Input: part model. Units: mm. Frame: model coordinates. A direction names the side the tool comes from. Give positions to 0.01 mm unless a question says otherwise; leave off trailing zeros. Write each loop counter-clockwise with the first axis right and the second up, starting at its lowest first coordinate (ties: lowest second). Pieces come first, ordered by that corner, then holes.
```python
from build123d import *

# Parameters (mm, degrees)
SKETCH_R        = 13
PAD_DEPTH       = 4
SKETCH001_R     = 11.2
SKETCH001_R_2   = 6.8
POCKET_DEPTH    = 0.5
SKETCH002_R     = 5
POCKET001_DEPTH = 8.001


with BuildPart() as part:
    # Sketch → Pad (new body, symmetric)
    with BuildSketch(Plane.XZ):
        Circle(SKETCH_R)
    extrude(amount=PAD_DEPTH, both=True)

    # Sketch001 (on Face2 of Pad) → Pocket (cut)
    with BuildSketch(Plane(origin=(0, 4, 0), x_dir=(1, 0, 0), z_dir=(0, 1, 0))):
        Circle(SKETCH001_R)
        Circle(SKETCH001_R_2, mode=Mode.SUBTRACT)
    pocket = extrude(amount=-POCKET_DEPTH, mode=Mode.SUBTRACT)

    # Mirrored: Pocket across XZ
    add(pocket.mirror(Plane.XZ), mode=Mode.SUBTRACT)

    # Sketch002 (on Face10 of Mirrored) → Pocket001 (cut, through all)
    with BuildSketch(Plane(origin=(0, 4, 0), x_dir=(1, 0, 0), z_dir=(0, 1, 0))):
        Circle(SKETCH002_R)
    extrude(amount=-POCKET001_DEPTH, mode=Mode.SUBTRACT)


solid = part.part
```
Item 1: Section B-B (z = 0). Return loops of the section in (x, y).
Item 2: Pin query (flat end, axial travel): pin 1 (5 mm diameter, centred on x = -0.5, z = 4, fed in from +Y); pin 2 (3 mm diameter, centred on y = 0.5, z = -7, fed in from +X); pin 3 (2 mm diameter, centred on x = -3, y = -1.5, fed in from +Z). Return the tip coordinate at first contact, or that it passes through.
Item 3: Section A-A (x = 0). Return loops of the section in (y, z), and give its area (3 significant figures).
Item 4: Ray query, line 1 (Z direction, x = 0, y = -3.55); line 2 (Z direction, x = 0, y = -0.5); line 3 (Y direction, x = -4.25, z = -9.75). Return the intervals inside material, ascending.
Item 5: Mould query, pull axis X, two halves, no side actions, for faces 1 (the flat face through (-4, -4, 4)), 2 (the flat face through (5, 3.5, 5)), 3 (the cylindrical face through (-10.316, -0.056, -7.91)). Classes: +X half, -X half, draft (parallel to the pull), parting line (faces both ways), or undercut.
Item 6: Set-up query: faces 4 (the cylindrical face through (-1.08, 0.06, 4.88)), 5 (the cylindrical face through (-1.47, 3.75, 6.64)), 6 (the cylindrical face through (-11.19, -3.75, -0.49)). Return all of +Z, -Z, +X, -X, +Y, -Y with unobstructed straight access to the full face (end or side cutting, diameter ignored); none if empty.
Item 7: Section C-C (z = 7.25). Return loops of the section in (x, y).
Item 8: Section D-D (y = 2.75). Return loops of the section in (x, z), and give its area (3 significant figures).
Solved:
1. outline: (-13, -4) - (-11.2, -4) - (-11.2, -3.5) - (-6.8, -3.5) - (-6.8, -4) - (-5, -4) - (-5, 4) - (-6.8, 4) - (-6.8, 3.5) - (-11.2, 3.5) - (-11.2, 4) - (-13, 4) - close; (5, -4) - (6.8, -4) - (6.8, -3.5) - (11.2, -3.5) - (11.2, -4) - (13, -4) - (13, 4) - (11.2, 4) - (11.2, 3.5) - (6.8, 3.5) - (6.8, 4) - (5, 4) - close
2. pin 1: stops at y = 4
2. pin 2: stops at x = 11.78
2. pin 3: stops at z = 12.85
3. outline: (-4, -13) - (4, -13) - (4, -11.2) - (3.5, -11.2) - (3.5, -6.8) - (4, -6.8) - (4, -5) - (-4, -5) - (-4, -6.8) - (-3.5, -6.8) - (-3.5, -11.2) - (-4, -11.2) - close; (-4, 5) - (4, 5) - (4, 6.8) - (3.5, 6.8) - (3.5, 11.2) - (4, 11.2) - (4, 13) - (-4, 13) - (-4, 11.2) - (-3.5, 11.2) - (-3.5, 6.8) - (-4, 6.8) - close
3. area: 119 mm2
4. line 1: z = -13 to -11.2, -6.8 to -5, 5 to 6.8, 11.2 to 13
4. line 2: z = -13 to -5, 5 to 13
4. line 3: y = -3.5 to 3.5
5. face 1: draft
5. face 2: undercut
5. face 3: parting line
6. face 4: +Y, -Y
6. face 5: +Y
6. face 6: -Y
7. outline: (-10.79, -4) - (-8.54, -4) - (-8.54, -3.5) - (8.54, -3.5) - (8.54, -4) - (10.79, -4) - (10.79, 4) - (8.54, 4) - (8.54, 3.5) - (-8.54, 3.5) - (-8.54, 4) - (-10.79, 4) - close
8. outline: circle Ø26 at (0, 0); hole circle Ø10 at (0, 0)
8. area: 452 mm2
